from build123d import *

# Parameters (mm, degrees)
SALIENTE_EXTRUIR1_DEPTH = 60
SALIENTE_EXTRUIR2_REACH = 64.405


with BuildPart() as part:
    # Croquis1 → Saliente-Extruir1 (new, symmetric)
    with BuildSketch(Plane.XY):
        Polygon((-0.25, -17), (-2.91801894, -17), (-10, 2), (-10, 14), (0, 14), (0, 0), (-6.586509369, 0), align=None)
    saliente_extruir1 = extrude(amount=SALIENTE_EXTRUIR1_DEPTH, both=True)

    # Saliente-Extruir2: up to this plane
    saliente_extruir2_end = Plane(origin=(-1, 0, 0), z_dir=(1, 0, 0))
    # Croquis2 → Saliente-Extruir2 (add, up to the surface)
    with BuildSketch(Plane(origin=(-5.783057557, -2.155552847, 0), x_dir=(0, 0, -1), z_dir=(0.9370248323365327, 0.3492627429095367, 0)), mode=Mode.PRIVATE) as saliente_extruir2_sk1:
        Polygon((-60, -12.842106464), (0, -12.842106464), (0, -10.842106464), (-4, -10.842106464), (-6.309401077, -10.842106464), (-14, -10.842106464), (-16.309401077, -10.842106464), (-24, -10.842106464), (-26.309401077, -10.842106464), (-34, -10.842106464), (-36.309401077, -10.842106464), (-44, -10.842106464), (-46.309401077, -10.842106464), (-54, -10.842106464), (-56.309401077, -10.842106464), (-60, -10.842106464), align=None)
    saliente_extruir2_tool1 = split(extrude(saliente_extruir2_sk1.sketch, amount=SALIENTE_EXTRUIR2_REACH, mode=Mode.PRIVATE), bisect_by=saliente_extruir2_end, keep=Keep.BOTH, mode=Mode.PRIVATE)
    # Croquis2 → Saliente-Extruir2 (add, up to the surface)
    with BuildSketch(Plane(origin=(-5.783057557, -2.155552847, 0), x_dir=(0, 0, -1), z_dir=(0.9370248323365327, 0.3492627429095367, 0)), mode=Mode.PRIVATE) as saliente_extruir2_sk2:
        Polygon((-60, -4.449801619), (-56.309401077, -10.842106464), (-54, -10.842106464), (-58.618802154, -2.842106464), (-60, -2.842106464), align=None)
    saliente_extruir2_tool2 = split(extrude(saliente_extruir2_sk2.sketch, amount=SALIENTE_EXTRUIR2_REACH, mode=Mode.PRIVATE), bisect_by=saliente_extruir2_end, keep=Keep.BOTH, mode=Mode.PRIVATE)
    # Croquis2 → Saliente-Extruir2 (add, up to the surface)
    with BuildSketch(Plane(origin=(-5.783057557, -2.155552847, 0), x_dir=(0, 0, -1), z_dir=(0.9370248323365327, 0.3492627429095367, 0)), mode=Mode.PRIVATE) as saliente_extruir2_sk3:
        Polygon((-26.309401077, -10.842106464), (-24, -10.842106464), (-28.618802154, -2.842106464), (-30.92820323, -2.842106464), align=None)
    saliente_extruir2_tool3 = split(extrude(saliente_extruir2_sk3.sketch, amount=SALIENTE_EXTRUIR2_REACH, mode=Mode.PRIVATE), bisect_by=saliente_extruir2_end, keep=Keep.BOTH, mode=Mode.PRIVATE)
    # Croquis2 → Saliente-Extruir2 (add, up to the surface)
    with BuildSketch(Plane(origin=(-5.783057557, -2.155552847, 0), x_dir=(0, 0, -1), z_dir=(0.9370248323365327, 0.3492627429095367, 0)), mode=Mode.PRIVATE) as saliente_extruir2_sk4:
        Polygon((-16.309401077, -10.842106464), (-14, -10.842106464), (-18.618802154, -2.842106464), (-20.92820323, -2.842106464), align=None)
    saliente_extruir2_tool4 = split(extrude(saliente_extruir2_sk4.sketch, amount=SALIENTE_EXTRUIR2_REACH, mode=Mode.PRIVATE), bisect_by=saliente_extruir2_end, keep=Keep.BOTH, mode=Mode.PRIVATE)
    # Croquis2 → Saliente-Extruir2 (add, up to the surface)
    with BuildSketch(Plane(origin=(-5.783057557, -2.155552847, 0), x_dir=(0, 0, -1), z_dir=(0.9370248323365327, 0.3492627429095367, 0)), mode=Mode.PRIVATE) as saliente_extruir2_sk5:
        Polygon((28.618802154, -2.842106464), (24, -10.842106464), (26.309401077, -10.842106464), (30.92820323, -2.842106464), align=None)
    saliente_extruir2_tool5 = split(extrude(saliente_extruir2_sk5.sketch, amount=SALIENTE_EXTRUIR2_REACH, mode=Mode.PRIVATE), bisect_by=saliente_extruir2_end, keep=Keep.BOTH, mode=Mode.PRIVATE)
    # Croquis2 → Saliente-Extruir2 (add, up to the surface)
    with BuildSketch(Plane(origin=(-5.783057557, -2.155552847, 0), x_dir=(0, 0, -1), z_dir=(0.9370248323365327, 0.3492627429095367, 0)), mode=Mode.PRIVATE) as saliente_extruir2_sk6:
        Polygon((34, -10.842106464), (36.309401077, -10.842106464), (40.92820323, -2.842106464), (38.618802154, -2.842106464), align=None)
    saliente_extruir2_tool6 = split(extrude(saliente_extruir2_sk6.sketch, amount=SALIENTE_EXTRUIR2_REACH, mode=Mode.PRIVATE), bisect_by=saliente_extruir2_end, keep=Keep.BOTH, mode=Mode.PRIVATE)
    # Croquis2 → Saliente-Extruir2 (add, up to the surface)
    with BuildSketch(Plane(origin=(-5.783057557, -2.155552847, 0), x_dir=(0, 0, -1), z_dir=(0.9370248323365327, 0.3492627429095367, 0)), mode=Mode.PRIVATE) as saliente_extruir2_sk7:
        Polygon((44, -10.842106464), (46.309401077, -10.842106464), (50.92820323, -2.842106464), (48.618802154, -2.842106464), align=None)
    saliente_extruir2_tool7 = split(extrude(saliente_extruir2_sk7.sketch, amount=SALIENTE_EXTRUIR2_REACH, mode=Mode.PRIVATE), bisect_by=saliente_extruir2_end, keep=Keep.BOTH, mode=Mode.PRIVATE)
    # Croquis2 → Saliente-Extruir2 (add, up to the surface)
    with BuildSketch(Plane(origin=(-5.783057557, -2.155552847, 0), x_dir=(0, 0, -1), z_dir=(0.9370248323365327, 0.3492627429095367, 0)), mode=Mode.PRIVATE) as saliente_extruir2_sk8:
        Polygon((54, -10.842106464), (56.309401077, -10.842106464), (60, -4.449801619), (60, -2.842106464), (58.618802154, -2.842106464), align=None)
    saliente_extruir2_tool8 = split(extrude(saliente_extruir2_sk8.sketch, amount=SALIENTE_EXTRUIR2_REACH, mode=Mode.PRIVATE), bisect_by=saliente_extruir2_end, keep=Keep.BOTH, mode=Mode.PRIVATE)
    # Croquis2 → Saliente-Extruir2 (add, up to the surface)
    with BuildSketch(Plane(origin=(-5.783057557, -2.155552847, 0), x_dir=(0, 0, -1), z_dir=(0.9370248323365327, 0.3492627429095367, 0)), mode=Mode.PRIVATE) as saliente_extruir2_sk9:
        Polygon((0, -12.842106464), (60, -12.842106464), (60, -10.842106464), (56.309401077, -10.842106464), (54, -10.842106464), (46.309401077, -10.842106464), (44, -10.842106464), (36.309401077, -10.842106464), (34, -10.842106464), (26.309401077, -10.842106464), (24, -10.842106464), (16.309401077, -10.842106464), (14, -10.842106464), (6.309401077, -10.842106464), (4, -10.842106464), (0, -10.842106464), align=None)
    saliente_extruir2_tool9 = split(extrude(saliente_extruir2_sk9.sketch, amount=SALIENTE_EXTRUIR2_REACH, mode=Mode.PRIVATE), bisect_by=saliente_extruir2_end, keep=Keep.BOTH, mode=Mode.PRIVATE)
    # Croquis2 → Saliente-Extruir2 (add, up to the surface)
    with BuildSketch(Plane(origin=(-5.783057557, -2.155552847, 0), x_dir=(0, 0, -1), z_dir=(0.9370248323365327, 0.3492627429095367, 0)), mode=Mode.PRIVATE) as saliente_extruir2_sk10:
        Polygon((-44, -10.842106464), (-48.618802154, -2.842106464), (-50.92820323, -2.842106464), (-46.309401077, -10.842106464), align=None)
    saliente_extruir2_tool10 = split(extrude(saliente_extruir2_sk10.sketch, amount=SALIENTE_EXTRUIR2_REACH, mode=Mode.PRIVATE), bisect_by=saliente_extruir2_end, keep=Keep.BOTH, mode=Mode.PRIVATE)
    # Croquis2 → Saliente-Extruir2 (add, up to the surface)
    with BuildSketch(Plane(origin=(-5.783057557, -2.155552847, 0), x_dir=(0, 0, -1), z_dir=(0.9370248323365327, 0.3492627429095367, 0)), mode=Mode.PRIVATE) as saliente_extruir2_sk11:
        Polygon((-34, -10.842106464), (-38.618802154, -2.842106464), (-40.92820323, -2.842106464), (-36.309401077, -10.842106464), align=None)
    saliente_extruir2_tool11 = split(extrude(saliente_extruir2_sk11.sketch, amount=SALIENTE_EXTRUIR2_REACH, mode=Mode.PRIVATE), bisect_by=saliente_extruir2_end, keep=Keep.BOTH, mode=Mode.PRIVATE)
    # Croquis2 → Saliente-Extruir2 (add, up to the surface)
    with BuildSketch(Plane(origin=(-5.783057557, -2.155552847, 0), x_dir=(0, 0, -1), z_dir=(0.9370248323365327, 0.3492627429095367, 0)), mode=Mode.PRIVATE) as saliente_extruir2_sk12:
        Polygon((-10.92820323, -2.842106464), (-6.309401077, -10.842106464), (-4, -10.842106464), (-8.618802154, -2.842106464), align=None)
    saliente_extruir2_tool12 = split(extrude(saliente_extruir2_sk12.sketch, amount=SALIENTE_EXTRUIR2_REACH, mode=Mode.PRIVATE), bisect_by=saliente_extruir2_end, keep=Keep.BOTH, mode=Mode.PRIVATE)
    # Croquis2 → Saliente-Extruir2 (add, up to the surface)
    with BuildSketch(Plane(origin=(-5.783057557, -2.155552847, 0), x_dir=(0, 0, -1), z_dir=(0.9370248323365327, 0.3492627429095367, 0)), mode=Mode.PRIVATE) as saliente_extruir2_sk13:
        Polygon((4, -10.842106464), (8.618802154, -2.842106464), (10.92820323, -2.842106464), (6.309401077, -10.842106464), align=None)
    saliente_extruir2_tool13 = split(extrude(saliente_extruir2_sk13.sketch, amount=SALIENTE_EXTRUIR2_REACH, mode=Mode.PRIVATE), bisect_by=saliente_extruir2_end, keep=Keep.BOTH, mode=Mode.PRIVATE)
    # Croquis2 → Saliente-Extruir2 (add, up to the surface)
    with BuildSketch(Plane(origin=(-5.783057557, -2.155552847, 0), x_dir=(0, 0, -1), z_dir=(0.9370248323365327, 0.3492627429095367, 0)), mode=Mode.PRIVATE) as saliente_extruir2_sk14:
        Polygon((14, -10.842106464), (18.618802154, -2.842106464), (20.92820323, -2.842106464), (16.309401077, -10.842106464), align=None)
    saliente_extruir2_tool14 = split(extrude(saliente_extruir2_sk14.sketch, amount=SALIENTE_EXTRUIR2_REACH, mode=Mode.PRIVATE), bisect_by=saliente_extruir2_end, keep=Keep.BOTH, mode=Mode.PRIVATE)
    saliente_extruir2 = saliente_extruir2_tool1.solids().sort_by_distance((-1.647051, -13.251901, 30))[0] + saliente_extruir2_tool2.solids().sort_by_distance((-3.342446, -8.703383, 57.344356))[0] + saliente_extruir2_tool3.solids().sort_by_distance((-3.393365, -8.566777, 27.464102))[0] + saliente_extruir2_tool4.solids().sort_by_distance((-3.393365, -8.566777, 17.464102))[0] + saliente_extruir2_tool5.solids().sort_by_distance((-3.393365, -8.566777, -27.464102))[0] + saliente_extruir2_tool6.solids().sort_by_distance((-3.393365, -8.566777, -37.464102))[0] + saliente_extruir2_tool7.solids().sort_by_distance((-3.393365, -8.566777, -47.464102))[0] + saliente_extruir2_tool8.solids().sort_by_distance((-3.342446, -8.703383, -57.344356))[0] + saliente_extruir2_tool9.solids().sort_by_distance((-1.647051, -13.251901, -30))[0] + saliente_extruir2_tool10.solids().sort_by_distance((-3.393365, -8.566777, 47.464102))[0] + saliente_extruir2_tool11.solids().sort_by_distance((-3.393365, -8.566777, 37.464102))[0] + saliente_extruir2_tool12.solids().sort_by_distance((-3.393365, -8.566777, 7.464102))[0] + saliente_extruir2_tool13.solids().sort_by_distance((-3.393365, -8.566777, -7.464102))[0] + saliente_extruir2_tool14.solids().sort_by_distance((-3.393365, -8.566777, -17.464102))[0]
    add(saliente_extruir2)

    # Simetría1: Saliente-Extruir1, Saliente-Extruir2 across plane
    add(saliente_extruir1.mirror(Plane(origin=(0, 0, 0), x_dir=(0, 0, 1), z_dir=(1, 0, 0))))
    add(saliente_extruir2.mirror(Plane(origin=(0, 0, 0), x_dir=(0, 0, 1), z_dir=(1, 0, 0))))


solid = part.part
Check sheet for the modelled part. Datum: model origin and axes. Units: mm. A direction names the side the tool comes from. Give positions to 0.01 mm unless a question says otherwise; leave off trailing zeros. Loops run counter-clockwise (first coordinate to the right, second up) from the corner with the lowest first, then second, coordinate; pieces in that order, holes last. Notation, with made-up numbers: M -11,33.25 L -7,33.25 A22 ccw -7,62.25 Z; hole C -8,23.25 d2. An arc over 180 degrees is marked long. Return JSON: item names as keys, results as strings. Group by question number.
1. Mould release check, pull along X, two halves, no side actions. Record for faces 1 (the flat face through (-10, 8, 1)), 2 (the flat face through (10, 8, 1)), 3 (the flat face through (2.92, -4.12, 49.76)), 4 (the flat face through (-2.24, -7.25, -39.1)): released by +X, released by -X, zero draft, split by the parting line, or undercut.
2. Thickness scan on L1, parallel to X at y = -14, z = -45; L2, parallel to X at y = -11, z = 21; L3, parallel to Y at x = 1.75, z = 1. Record the ranges inside material, lowest first.
3. Cross-section at A-A on y = -2. Record the boundary of the cut face in (x, z).
4. Tool access check on faces 5 (the flat face through (2.14, -8.15, 58.59)), 6 (the flat face through (-2.24, -7.25, -16.79)), 7 (the flat face through (-6.41, -7.63, 0.84)), 8 (the flat face through (-2.92, -4.12, -29.79)). Record the directions out of +Z, -Z, +X, -X, +Y, -Y that give a thin tool (end or side, any length) a straight path to the whole face; none if there is none.
5. Go/stop test with flat-tipped pins: pin 1 (3 mm diameter, centred on y = -9.5, z = -17.5, fed in from +X); pin 2 (8.5 mm diameter, centred on y = -10, z = 3, fed in from -X); pin 3 (1.5 mm diameter, centred on y = -13.5, z = -42, fed in from -X). Record where each tip stops, or that it passes through.
Return value:
{
 "1": {"face 1": "released by -X", "face 2": "released by +X", "face 3": "undercut", "face 4": "undercut"},
 "2": {"L1": "-4.04 to -1, 1 to 4.04", "L2": "-5.15 to -2.49, 2.49 to 5.15", "L3": "-17 to -12.22, 0 to 14"},
 "3": {"outline": "M -8.51,-60 L -5.84,-60 L -5.84,60 L -8.51,60 Z; M 5.84,-60 L 8.51,-60 L 8.51,60 L 5.84,60 Z"},
 "4": {"face 5": "+Z", "face 6": "none", "face 7": "+Z, -Z, -X, -Y", "face 8": "+Z, -Z"},
 "5": {"pin 1": "x = 6.27", "pin 2": "x = -7.11", "pin 3": "x = -4.5"}
}
